For this review, take the finished solid that the model builds, in its own axes (mm). Give positions to 0.01 mm unless a question says otherwise; leave off trailing zeros. Write each loop counter-clockwise with the first axis right and the second up, starting at its lowest first coordinate (ties: lowest second). Pieces come first, ordered by that corner, then holes.
from build123d import *

# Parameters (mm, degrees)
SKETCH2_W           = 20
SKETCH2_H           = 15
BOSS_EXTRUDE1_DEPTH = 5
SKETCH3_R           = 1.6
CUT_EXTRUDE1_DEPTH  = 6
FILLET1_R           = 2


with BuildPart() as part:
    # Sketch2 → Boss-Extrude1 (new body)
    with BuildSketch(Plane(origin=(0, 0, 0), x_dir=(1, 0, 0), z_dir=(0, 1, 0))):
        with Locations((10, 7.5)):
            Rectangle(SKETCH2_W, SKETCH2_H)
    extrude(amount=BOSS_EXTRUDE1_DEPTH)

    # Sketch3 → Cut-Extrude1 (cut, through all)
    with BuildSketch(Plane(origin=(0, 5, 0), x_dir=(1, 0, 0), z_dir=(0, 1, 0))):
        with Locations((10, 7.5)):
            Circle(SKETCH3_R)
    extrude(amount=-CUT_EXTRUDE1_DEPTH, mode=Mode.SUBTRACT)

    # Fillet1
    fillet1_edges = [part.edges().sort_by_distance(p)[0] for p in [
        (10, 5, -15),
        (0, 5, -7.5),
        (10, 5, 0),
        (0, 2.5, 0),
        (0, 2.5, -15),
        (20, 2.5, -15),
        (20, 2.5, 0),
        (20, 5, -7.5),
    ]]
    fillet(fillet1_edges, radius=FILLET1_R)


solid = part.part
(1) The part is to be moulded in two halves that separate along X. For faces 1 (the flat face through (9.9, 0, -9.3)), 2 (the cylindrical face through (19.4, 4.43, -7.58)), 3 (the cylindrical face through (8.73, 2.54, -6.53)), 4 (the cylindrical face through (0.57, 1.52, -0.6)), say which applies: +X half, -X half, draft (parallel to the pull), parting line (faces both ways), or undercut.
(2) Clearance check with a flat-ended pin moving along its axis: pin 1 Ø1.9 at (x, z) = (10, -7.5) entering from -Y. State where the tip first meets the part, or that it passes through.
(3) We need section B-B (z = -6.5). Write out the cut boundary in (x, y), and give its area (3 significant figures).
(4) For L1, parallel to Z at x = 10, y = 2.65; L2, parallel to X at y = 0.95, z = -7.5; L3, parallel to Z at x = 11, y = 4.4, list the stretches that pass through material, from the lowest coordinate up.
(5) We need section C-C (y = 2.65). Write out the cut boundary in (x, z), and give its area (3 significant figures).
(6) We need section A-A (x = 10). Write out the cut boundary in (y, z).
(7) We need section D-D (x = 15.5). Write out the cut boundary in (y, z).
The answers:
1. face 1: draft
1. face 2: +X half
1. face 3: undercut
1. face 4: -X half
2. pin 1: passes through
3. outline: (0, 0) - (8.75, 0) - (8.75, 5) - (2, 5) arc R2 ccw to (0, 3) - close; (11.25, 0) - (20, 0) - (20, 3) arc R2 ccw to (18, 5) - (11.25, 5) - close
3. area: 85.8 mm2
4. L1: z = -15 to -9.1, -5.9 to 0
4. L2: x = 0 to 8.4, 11.6 to 20
4. L3: z = -14.43 to -8.75, -6.25 to -0.57
5. outline: (0, -13) arc R2 ccw to (2, -15) - (18, -15) arc R2 ccw to (20, -13) - (20, -2) arc R2 ccw to (18, 0) - (2, 0) arc R2 ccw to (0, -2) - close; hole circle Ø3.2 at (10, -7.5)
5. area: 289 mm2
6. outline: (0, -15) - (3, -15) arc R2 ccw to (5, -13) - (5, -9.1) - (0, -9.1) - close; (0, -5.9) - (5, -5.9) - (5, -2) arc R2 ccw to (3, 0) - (0, 0) - close
7. outline: (0, -15) - (3, -15) arc R2 ccw to (5, -13) - (5, -2) arc R2 ccw to (3, 0) - (0, 0) - close
